For this review, take the finished solid that the model builds, in its own axes (mm). A direction names the side the tool comes from. Round coordinates to 2 decimals unless told otherwise and drop trailing zeros. Order: outer loops, then holes, each group sorted by start corner. A loop starts at its lowest first (then second) coordinate and runs counter-clockwise, first axis right, second up. Notation, with made-up numbers: M 18,18 L 24,18 A30 cw 24,42 Z; hole C -17,-38 d10. An arc over 180 degrees is marked long. Put each result on its own line as item: value.
from build123d import *

# Parameters (mm, degrees)
BOSS_EXTRUDE1_DEPTH  = 19.75
SKETCH2_W            = 28
SKETCH2_H            = 5
CUT_EXTRUDE1_DEPTH   = 39.25
SKETCH3_W            = 6
SKETCH3_H            = 5
BOSS_EXTRUDE2_DEPTH  = 4
BOSS_EXTRUDE4_DEPTH  = 5
BOSS_EXTRUDE5_START  = -5
BOSS_EXTRUDE5_DEPTH  = 5
CHAMFER2_SIZE        = 2
FILLET1_R            = 2
CUT_EXTRUDE3_DEPTH   = 42.337785379
BOSS_EXTRUDE6_DEPTH  = 6
FILLET2_R            = 1.5
SKETCH11_R           = 2.5
SKETCH11_R_2         = 1
BOSS_EXTRUDE7_DEPTH  = 10.5
FILLET3_R            = 1
FILLET4_R            = 1.5
SKETCH13_W           = 6
SKETCH13_H           = 7
BOSS_EXTRUDE8_DEPTH  = 2.5
SKETCH14_R           = 1.2
CUT_EXTRUDE6_DEPTH   = 42.237877006
BOSS_EXTRUDE9_DEPTH  = 2.5
FILLET5_R            = 2
SKETCH18_W           = 1.5
SKETCH18_H           = 1.5
BOSS_EXTRUDE10_DEPTH = 0.75
SKETCH19_W           = 1.5
SKETCH19_H           = 1.5
BOSS_EXTRUDE11_DEPTH = 0.75


with BuildPart() as part:
    # Sketch1 → Boss-Extrude1 (new, symmetric)
    with BuildSketch(Plane.XY):
        Polygon((-25, 24), (32, 24), (32, 22.5), (-23.5, 22.5), (-23.5, 15.5), (-26.5, 15.5), (-26.5, 17), (-25, 17), align=None)
    extrude(amount=BOSS_EXTRUDE1_DEPTH, both=True)

    # Sketch2 → Cut-Extrude1 (cut, through all)
    with BuildSketch(Plane.XZ.offset(-22.5)):
        with Locations((0, 17.25)):
            Rectangle(SKETCH2_W, SKETCH2_H)
        with Locations((0, -17.25)):
            Rectangle(SKETCH2_W, SKETCH2_H)
    extrude(amount=-CUT_EXTRUDE1_DEPTH, mode=Mode.SUBTRACT)

    # Sketch3 → Boss-Extrude2 (add)
    with BuildSketch(Plane(origin=(0, 24, 0), x_dir=(1, 0, 0), z_dir=(0, 1, 0))):
        with Locations((-17, 22.25)):
            Rectangle(SKETCH3_W, SKETCH3_H)
        with Locations((17, 22.25)):
            Rectangle(SKETCH3_W, SKETCH3_H)
        with Locations((17, -22.25)):
            Rectangle(SKETCH3_W, SKETCH3_H)
        with Locations((-17, -22.25)):
            Rectangle(SKETCH3_W, SKETCH3_H)
    extrude(amount=-BOSS_EXTRUDE2_DEPTH)

    # Sketch6 → Boss-Extrude4 (add)
    with BuildSketch(Plane(origin=(0, 0, -24.75), x_dir=(-1, 0, 0), z_dir=(0, 0, -1))):
        with BuildLine():
            Line((20, 24), (25, 24))
            Line((25, 24), (25, 15.5))
            Line((25, 15.5), (23.5, 15.5))
            Line((23.5, 15.5), (22.25, 16.75))
            Line((22.25, 16.75), (22.25, 17))
            ThreePointArc((22.25, 17), (21.371320344, 19.121320344), (19.25, 20))
            Line((19.25, 20), (20, 20))
            Line((20, 20), (20, 24))
        make_face()
    extrude(amount=-BOSS_EXTRUDE4_DEPTH)

    # Sketch7 → Boss-Extrude5 (add)
    with BuildSketch(Plane.XY.offset(24.75).offset(BOSS_EXTRUDE5_START)):
        with BuildLine():
            Line((-20, 20), (-20, 24))
            Line((-20, 24), (-25, 24))
            Line((-25, 24), (-25, 15.5))
            Line((-25, 15.5), (-23.5, 15.5))
            Line((-23.5, 15.5), (-22.25, 16.75))
            Line((-22.25, 16.75), (-22.25, 17))
            ThreePointArc((-22.25, 17), (-21.371320344, 19.121320344), (-19.25, 20))
            Line((-19.25, 20), (-20, 20))
        make_face()
    extrude(amount=BOSS_EXTRUDE5_DEPTH)

    # Chamfer2
    chamfer2_edges = [part.edges().sort_by_distance(p)[0] for p in [
        (-25, 19.75, -24.75),
        (-25, 19.75, 24.75),
    ]]
    chamfer(chamfer2_edges, length=CHAMFER2_SIZE)

    # Fillet1
    fillet1_edges = [part.edges().sort_by_distance(p)[0] for p in [
        (14, 23.25, 14.75),
        (-14, 23.25, 14.75),
        (-14, 23.25, -14.75),
        (14, 23.25, -14.75),
        (14, 22, 24.75),
        (20, 23.25, 19.75),
        (20, 22, 24.75),
        (-14, 22, 24.75),
        (20, 23.25, -19.75),
        (14, 22, -24.75),
        (20, 22, -24.75),
        (-14, 22, -24.75),
    ]]
    fillet(fillet1_edges, radius=FILLET1_R)

    # Sketch8 → Cut-Extrude3 (cut, through all)
    with BuildSketch(Plane(origin=(0, 24, 0), x_dir=(1, 0, 0), z_dir=(0, 1, 0))):
        Polygon((-25, 17.5), (-22, 17.5), (-22, -17.5), (-25, -17.5), (-26.867861181, -17.5), (-26.867861181, 17.5), align=None)
    extrude(amount=-CUT_EXTRUDE3_DEPTH, mode=Mode.SUBTRACT)

    # Sketch9 → Boss-Extrude6 (add)
    with BuildSketch(Plane.XZ.offset(-15.5)):
        Polygon((-25, 22.75), (-29, 18.75), (-29, 17.5), (-26.5, 17.5), (-26.5, 20.5), (-25, 20.5), align=None)
        Polygon((-25, -20.5), (-25, -22.75), (-29, -18.75), (-29, -17.5), (-26.5, -17.5), (-26.5, -20.5), align=None)
    extrude(amount=-BOSS_EXTRUDE6_DEPTH)

    # Fillet2
    fillet2_edges = [part.edges().sort_by_distance(p)[0] for p in [
        (-25, 21.5, 21.625),
        (-25, 21.5, -21.625),
    ]]
    fillet(fillet2_edges, radius=FILLET2_R)

    # Sketch11 → Boss-Extrude7 (add)
    # profile 1 of 2: a face of its own
    with BuildSketch(Plane.XZ.offset(-22.5)):
        with Locations(Location((10, 0, 0), (0, 0, 90))):
            Circle(SKETCH11_R)
        with Locations(Location((10, 0, 0), (0, 0, 90))):
            Circle(SKETCH11_R_2, mode=Mode.SUBTRACT)
    # profile 2 of 2: a face of its own
    with BuildSketch(Plane.XZ.offset(-22.5)):
        with Locations(Location((-10, 0, 0), (0, 0, 90))):
            Circle(SKETCH11_R)
        with Locations(Location((-10, 0, 0), (0, 0, 90))):
            Circle(SKETCH11_R_2, mode=Mode.SUBTRACT)
    extrude(amount=BOSS_EXTRUDE7_DEPTH)

    # Fillet3
    fillet3_edges = [part.edges().sort_by_distance(p)[0] for p in [
        (10, 22.5, -2.5),
        (-10, 22.5, -2.5),
    ]]
    fillet(fillet3_edges, radius=FILLET3_R)

    # Fillet4
    fillet4_edges = [part.edges().sort_by_distance(p)[0] for p in [
        (32, 23.25, -19.75),
        (32, 23.25, 19.75),
        (-22, 23.25, -17.5),
        (-22, 23.25, 17.5),
    ]]
    fillet(fillet4_edges, radius=FILLET4_R)

    # Sketch13 → Boss-Extrude8 (add)
    with BuildSketch(Plane.XZ.offset(-22.5)):
        with Locations((17, 16.25)):
            Rectangle(SKETCH13_W, SKETCH13_H)
        with Locations((17, -16.25)):
            Rectangle(SKETCH13_W, SKETCH13_H)
        with Locations((-17, -16.25)):
            Rectangle(SKETCH13_W, SKETCH13_H)
        with Locations((-17, 16.25)):
            Rectangle(SKETCH13_W, SKETCH13_H)
    extrude(amount=BOSS_EXTRUDE8_DEPTH)

    # Sketch14 → Cut-Extrude6 (cut, through all)
    with BuildSketch(Plane.XZ.offset(-20)):
        with Locations((16, 19.75)):
            Circle(SKETCH14_R)
        with Locations(Location((-16, 19.75, 0), (0, 0, 180))):
            Circle(SKETCH14_R)
        with Locations((-16, -19.75)):
            Circle(SKETCH14_R)
        with Locations(Location((16, -19.75, 0), (0, 0, 180))):
            Circle(SKETCH14_R)
    extrude(amount=-CUT_EXTRUDE6_DEPTH, mode=Mode.SUBTRACT)

    # Sketch15 → Boss-Extrude9 (add)
    with BuildSketch(Plane.XZ.offset(-22.5)):
        with BuildLine():
            Line((14, 16.75), (14, 12.75))
            Line((14, 12.75), (-14, 12.75))
            Line((-14, 12.75), (-14, 16.75))
            ThreePointArc((-14, 16.75), (-13.414213562, 15.335786438), (-12, 14.75))
            Line((-12, 14.75), (12, 14.75))
            ThreePointArc((12, 14.75), (13.414213562, 15.335786438), (14, 16.75))
        make_face()
        with BuildLine():
            Line((-14, -12.75), (14, -12.75))
            Line((14, -12.75), (14, -16.75))
            ThreePointArc((14, -16.75), (13.414213562, -15.335786438), (12, -14.75))
            Line((12, -14.75), (-12, -14.75))
            ThreePointArc((-12, -14.75), (-13.414213562, -15.335786438), (-14, -16.75))
            Line((-14, -16.75), (-14, -12.75))
        make_face()
    extrude(amount=BOSS_EXTRUDE9_DEPTH)

    # Fillet5
    fillet5_edges = [part.edges().sort_by_distance(p)[0] for p in [
        (20, 21.25, 12.75),
        (20, 21.25, -12.75),
        (-20, 21.25, -12.75),
        (-20, 21.25, 12.75),
    ]]
    fillet(fillet5_edges, radius=FILLET5_R)

    # Sketch18 → Boss-Extrude10 (add)
    with BuildSketch(Plane.XY.offset(19.75)):
        with Locations((-25.75, 16.25)):
            Rectangle(SKETCH18_W, SKETCH18_H)
    extrude(amount=BOSS_EXTRUDE10_DEPTH)

    # Sketch19 → Boss-Extrude11 (add)
    with BuildSketch(Plane(origin=(0, 0, -19.75), x_dir=(-1, 0, 0), z_dir=(0, 0, -1))):
        with Locations((25.75, 16.25)):
            Rectangle(SKETCH19_W, SKETCH19_H)
    extrude(amount=BOSS_EXTRUDE11_DEPTH)


solid = part.part
(1) Add section D-D on z = -8. Give the boundary of the cut face in (x, y).
A:
outline: M -22,22.5 L 32,22.5 L 32,24 L -22,24 Z
(2) Draft analysis for pull direction X (two halves, no side actions). For faces 6 (the face through (0, 21, -12.75)), 7 (the face through (-23, 16, -22)), 8 (the face through (14.57, 21.97, -24.15)), 9 (the face through (-19.4, 21.23, 13.32)), state which applies: released by +X, released by -X, zero draft, split by the parting line, or undercut.
A:
face 6: zero draft
face 7: released by +X
face 8: undercut
face 9: released by -X
(3) Insertion check: pin 1 Ø3 at (x, z) = (23, -13) entering from -Y; pin 2 Ø1.5 at (y, z) = (20.5, -16) entering from +X; pin 3 Ø1.6 at (y, z) = (20.5, -21) entering from -X. Each pin has a flat end and moves straight along its axis. Give the tip position at first contact, or say it passes through.
A:
pin 1: stops at y = 22.5
pin 2: stops at x = 20
pin 3: stops at x = -27.55
(4) For faces 1 (the face through (-22, 23, 0)), 2 (the face through (9, 17, 0)), 3 (the face through (14, 22, -20)), 4 (the face through (26, 23, -19.75)), 5 (the face through (-25, 21, 19)), list the 3-axis set-ups (+Z, -Z, +X, -X, +Y, -Y) from which the entire face can be reached by the end or side of a thin tool; tool diameter is ignored.
A:
face 1: -X, +Y, -Y
face 2: -Y
face 3: -Z, +Y, -Y
face 4: -Z, +X, +Y, -Y
face 5: +Y
(5) To check wall thickness, follow L1, parallel to X at y = 18, z = 0; L2, parallel to Z at x = -16, y = 23; L3, parallel to Z at x = 16, y = 21.1. State the ranges of each line that lie inside material, in increasing order.
A:
L1: x = -12.5 to -11, -9 to -7.5, 7.5 to 9, 11 to 12.5
L2: z = -24.75 to -20.95, -18.55 to 18.55, 20.95 to 24.75
L3: z = -24.75 to -20.95, -18.55 to -12.75, 12.75 to 18.55, 20.95 to 24.75
(6) Add section C-C on x = -10. Give the boundary of the cut face in (y, z).
A:
outline: M 12,-2.5 L 21.5,-2.5 A1 cw 22.5,-3.5 L 22.5,-12.75 L 20,-12.75 L 20,-14.75 L 24,-14.75 L 24,14.75 L 20,14.75 L 20,12.75 L 22.5,12.75 L 22.5,3.5 A1 cw 21.5,2.5 L 12,2.5 L 12,1 L 22.5,1 L 22.5,-1 L 12,-1 Z
(7) Add section B-B on z = 0. Give the boundary of the cut face in (x, y), then the cut area to 3 significant figures.
A:
outline: M -22,22.5 L -13.5,22.5 A1 cw -12.5,21.5 L -12.5,12 L -11,12 L -11,22.5 L -9,22.5 L -9,12 L -7.5,12 L -7.5,21.5 A1 cw -6.5,22.5 L 6.5,22.5 A1 cw 7.5,21.5 L 7.5,12 L 9,12 L 9,22.5 L 11,22.5 L 11,12 L 12.5,12 L 12.5,21.5 A1 cw 13.5,22.5 L 32,22.5 L 32,24 L -22,24 Z
area: 145 mm2
(8) Add section A-A on y = 13. Give the boundary of the cut face in (x, z).
A:
outline: C -10,0 d5; C 10,0 d5; hole C -10,0 d2; hole C 10,0 d2
